```python
from build123d import *

# Parameters (mm, degrees)
SKETCH1_W           = 500
SKETCH1_H           = 500
BOSS_EXTRUDE1_DEPTH = 6.35
SKETCH2_R           = 84
CUT_EXTRUDE1_DEPTH  = 6.35
CUT_EXTRUDE2_DEPTH  = 6.35
FILLET1_R           = 15


with BuildPart() as part:
    # Sketch1 → Boss-Extrude1 (new body)
    with BuildSketch(Plane(origin=(0, 0, 0), x_dir=(1, 0, 0), z_dir=(0, 1, 0))):
        with Locations((20.161290323, -38.306451613)):
            Rectangle(SKETCH1_W, SKETCH1_H)
    extrude(amount=BOSS_EXTRUDE1_DEPTH)

    # Sketch2 → Cut-Extrude1 (cut)
    with BuildSketch(Plane(origin=(0, 6.35, 0), x_dir=(1, 0, 0), z_dir=(0, 1, 0))):
        with Locations(Location((20.161290323, -38.306451613, 0), (0, 0, 270))):
            Circle(SKETCH2_R)
    extrude(amount=-CUT_EXTRUDE1_DEPTH, mode=Mode.SUBTRACT)

    # Sketch3 → Cut-Extrude2 (cut)
    with BuildSketch(Plane(origin=(0, 6.35, 0), x_dir=(1, 0, 0), z_dir=(0, 1, 0))):
        with BuildLine():
            Line((-38.161167808, 9.435852288), (-27.555823691, 20.043711457))
            add(Edge.make_bspline(
                [(-38.161167808, 9.435852288), (-209.678686167, 191.47297422), (-27.555823691, 20.043711457)],
                knots=[0, 0, 0, 1, 1, 1], degree=2, weights=[1, 0.436781609, 1]))
        make_face()
        with BuildLine():
            Line((-27.581013578, -96.628911245), (-38.188872748, -86.023567127))
            add(Edge.make_bspline(
                [(-27.581013578, -96.628911245), (-209.61813551, -268.146429603), (-38.188872748, -86.023567127)],
                knots=[0, 0, 0, 1, 1, 1], degree=2, weights=[1, 0.436781609, 1]))
        make_face()
        with BuildLine():
            Line((78.483749955, -86.048757015), (67.878405837, -96.656616184))
            add(Edge.make_bspline(
                [(78.483749955, -86.048757015), (250.001268313, -268.085878946), (67.878405837, -96.656616184)],
                knots=[0, 0, 0, 1, 1, 1], degree=2, weights=[1, 0.436781609, 1]))
        make_face()
        with BuildLine():
            Line((67.903595725, 20.016006518), (78.511454894, 9.410662401))
            add(Edge.make_bspline(
                [(67.903595725, 20.016006518), (249.940717656, 191.533524877), (78.511454894, 9.410662401)],
                knots=[0, 0, 0, 1, 1, 1], degree=2, weights=[1, 0.436781609, 1]))
        make_face()
    extrude(amount=-CUT_EXTRUDE2_DEPTH, mode=Mode.SUBTRACT)

    # Fillet1
    fillet1_edges = [part.edges().sort_by_distance(p)[0] for p in [
        (-33.927432607, 3.175, 102.574717902),
        (-44.128484725, 3.175, 92.369607499),
        (84.429555949, 3.175, 92.395175331),
        (74.224445361, 3.175, 102.596227373),
        (-44.106975254, 3.175, -15.782272163),
        (-33.901864775, 3.175, -25.983324098),
        (74.250014887, 3.175, -25.961813301),
        (84.451066746, 3.175, -15.756702637),
    ]]
    fillet(fillet1_edges, radius=FILLET1_R)


solid = part.part
```
Geometry: final body of the model. Coordinates: model frame, mm. A direction names the side the tool comes from. Round coordinates to 2 decimals unless told otherwise and drop trailing zeros. Loops run counter-clockwise (first coordinate to the right, second up) from the corner with the lowest first, then second, coordinate; pieces in that order, holes last.
Item 1: Section C-C, the plane z = -58. State how many separate pieces and enclosed holes the cut face has, plus the area to 3 significant figures.
Checked values:
separate pieces: 3
enclosed holes: 0
area: 3,040 mm2
Item 2: Contact query for a flat-ended pin moving along its axis: P1, Ø2, axis at x = 103.5, z = 14, coming from the -Y side. Output: stop coordinate, or through.
Checked values:
P1: stops at y = 0
Item 3: Reachability of faces 3 (the flat face through (-94, 6.35, 35)), 4 (the cylindrical face through (-63.836, 3.219, 37.631)) from +Z, -Z, +X, -X, +Y, -Y: full face, straight path, thin tool, end or side. Return the list, or none.
Checked values:
face 3: +Z, -Z, +X, -X, +Y
face 4: +Y, -Y
Item 4: Section B-B, the plane x = 13. Output: boundary loops of the cut face in (y, z).
Checked values:
outline: (0, -211.69) - (6.35, -211.69) - (6.35, -45.39) - (0, -45.39) - close; (0, 122) - (6.35, 122) - (6.35, 288.31) - (0, 288.31) - close
Item 5: Mould query, pull axis X, two halves, no side actions, for faces 1 (the cylindrical face through (104.16, 3.22, 38.98)), 2 (the flat face through (-94, 0, 35)). Classes: released by +X, released by -X, zero draft, split by the parting line, or undercut.
Checked values:
face 1: undercut
face 2: zero draft
Item 6: Section A-A, the plane z = 11. Output: boundary loops of the cut face in (x, y).
Checked values:
outline: (-229.84, 0) - (-59.28, 0) - (-59.28, 6.35) - (-229.84, 6.35) - close; (99.6, 0) - (270.16, 0) - (270.16, 6.35) - (99.6, 6.35) - close
Item 7: Line query: L1, parallel to X at y = 1, z = -33; L2, parallel to X at y = 1, z = 34; L3, parallel to Z at x = 126.5, y = 3.5. Output: solid intervals per line, ascending.
Checked values:
L1: x = -229.84 to -59.84, -41.29 to -24.24, 64.56 to 81.66, 100.19 to 270.16
L2: x = -229.84 to -63.73, 104.05 to 270.16
L3: z = -211.69 to -68.64, -65.97 to 142.59, 145.26 to 288.31
